Geometry: final body of the model. Coordinates: model frame, mm. A direction names the side the tool comes from. Give positions to 0.01 mm unless a question says otherwise; leave off trailing zeros. Write each loop counter-clockwise with the first axis right and the second up, starting at its lowest first coordinate (ties: lowest second). Pieces come first, ordered by that corner, then holes. Notation, with made-up numbers: M -24,15 L 21,15 A22 cw 21,47 Z; hole C 7,-4 d1. An arc over 180 degrees is marked long. Answer as a JSON object with one key per item and string values.
from build123d import *

# Parameters (mm, degrees)
EXTRUDE_1_DEPTH    = 10.5
HOLE_WIZARD_M8_1_D = 6.8


with BuildPart() as part:
    # 草图1 → 凸台-拉伸1 (new, symmetric)
    with BuildSketch(Plane.XY):
        with BuildLine():
            Line((-3.7, 0), (3.7, 0))
            ThreePointArc((3.7, 0), (3.912132034, 0.087867966), (4, 0.3))
            Line((4, 0.3), (4, 0.5))
            ThreePointArc((4, 0.5), (4.087867966, 0.712132034), (4.3, 0.8))
            Line((4.3, 0.8), (6.25, 0.8))
            ThreePointArc((6.25, 0.8), (6.462132034, 0.887867966), (6.55, 1.1))
            Line((6.55, 1.1), (6.55, 1.214694733))
            ThreePointArc((6.55, 1.214694733), (6.538468452, 1.297071625), (6.504760317, 1.37311563))
            ThreePointArc((6.504760317, 1.37311563), (3.934117906, 4.65105617), (0.716844819, 7.297232748))
            ThreePointArc((0.716844819, 7.297232748), (0, 7.6), (-0.716844819, 7.297232748))
            ThreePointArc((-0.716844819, 7.297232748), (-3.934117906, 4.65105617), (-6.504760317, 1.37311563))
            ThreePointArc((-6.504760317, 1.37311563), (-6.538468452, 1.297071625), (-6.55, 1.214694733))
            Line((-6.55, 1.214694733), (-6.55, 1.1))
            ThreePointArc((-6.55, 1.1), (-6.462132034, 0.887867966), (-6.25, 0.8))
            Line((-6.25, 0.8), (-4.3, 0.8))
            ThreePointArc((-4.3, 0.8), (-4.087867966, 0.712132034), (-4, 0.5))
            Line((-4, 0.5), (-4, 0.3))
            ThreePointArc((-4, 0.3), (-3.912132034, 0.087867966), (-3.7, 0))
        make_face()
    extrude(amount=EXTRUDE_1_DEPTH, both=True)

    # M8 螺纹孔1 (through all)
    with Locations(Plane(origin=(0, 0, -4), x_dir=(0, 0, -1), z_dir=(0, -1, 0))):
        with Locations((0, 0)):
            Hole(HOLE_WIZARD_M8_1_D / 2)


solid = part.part
1) Line query: line 1 (Z direction, x = 0, y = 2); line 2 (Z direction, x = 1, y = 6.5); line 3 (X direction, y = 2.5, z = -5). Output: solid intervals per line, ascending. Write a range as from..to.
Geometry check:
{"line 1": "z = -10.5..-7.4, -0.6..10.5", "line 2": "z = -10.5..-7.25, -0.75..10.5", "line 3": "x = -5.75..-3.25, 3.25..5.75"}
2) Cut plane A-A on x = 0. Return loops of the section in (y, z), and give its area (3 significant figures).
Geometry check:
{"outline": "M 0,-10.5 L 7.6,-10.5 L 7.6,-7.4 L 0,-7.4 Z; M 0,-0.6 L 7.6,-0.6 L 7.6,10.5 L 0,10.5 Z", "area": "108 mm2"}
3) Contact query for flat-ended pins moving along their axis: P1, Ø6, axis at x = 0, z = -4, coming from the +Y side; P2, Ø0.6, axis at x = -5.5, z = -2, coming from the -Y side; P3, Ø4, axis at y = 3.5, z = 4.5, coming from the -X side. Output: stop coordinate, or through.
Geometry check:
{"P1": "passes through", "P2": "stops at y = 0.8", "P3": "stops at x = -6.43"}
4) Cut plane B-B on y = 6.5. Return loops of the section in (x, z), and give its area (3 significant figures).
Geometry check:
{"outline": "M -1.84,-10.5 L 1.84,-10.5 L 1.84,-6.86 A3.4 cw -1.84,-6.86 Z; M -1.84,-1.14 A3.4 cw 1.84,-1.14 L 1.84,10.5 L -1.84,10.5 Z", "area": "53.7 mm2"}
5) Set-up query: faces 1 (the cylindrical face through (0, 7.6, 5)), 2 (the flat face through (-5, 0.8, 0)), 3 (the flat face through (5, 0.8, 0)). Return all of +Z, -Z, +X, -X, +Y, -Y with unobstructed straight access to the full face (end or side cutting, diameter ignored); none if empty.
Geometry check:
{"face 1": "+Z, -Z, +Y", "face 2": "+Z, -Z, -X, -Y", "face 3": "+Z, -Z, +X, -Y"}
6) Cut plane C-C on z = -4. Return loops of the section in (x, y), and give its area (3 significant figures).
Geometry check:
{"outline": "M -6.55,1.1 A0.3 ccw -6.25,0.8 L -4.3,0.8 A0.3 cw -4,0.5 L -4,0.3 A0.3 ccw -3.7,0 L -3.4,0 L -3.4,5.18 A19.2 ccw -6.5,1.37 A0.3 ccw -6.55,1.21 Z; M 3.4,0 L 3.7,0 A0.3 ccw 4,0.3 L 4,0.5 A0.3 cw 4.3,0.8 L 6.25,0.8 A0.3 ccw 6.55,1.1 L 6.55,1.21 A0.3 ccw 6.5,1.37 A19.2 ccw 3.4,5.18 Z", "area": "17.4 mm2"}
7) Cut plane D-D on z = 5.25. Return loops of the section in (x, y), and give its area (3 significant figures).
Geometry check:
{"outline": "M -6.55,1.1 A0.3 ccw -6.25,0.8 L -4.3,0.8 A0.3 cw -4,0.5 L -4,0.3 A0.3 ccw -3.7,0 L 3.7,0 A0.3 ccw 4,0.3 L 4,0.5 A0.3 cw 4.3,0.8 L 6.25,0.8 A0.3 ccw 6.55,1.1 L 6.55,1.21 A0.3 ccw 6.5,1.37 A19.2 ccw 0.72,7.3 A1 ccw -0.72,7.3 A19.2 ccw -6.5,1.37 A0.3 ccw -6.55,1.21 Z", "area": "61.9 mm2"}
